The model under review builds one solid part; all positions refer to its coordinate system, in mm. A direction names the side the tool comes from. Coordinates: 2 decimals unless noted, no trailing zeros. Order: outer loops, then holes, each group sorted by start corner. A loop starts at its lowest first (then second) coordinate and runs counter-clockwise, first axis right, second up. Notation, with made-up numbers: M -6.5,58 L 32.5,58 A38 ccw 32.5,97 Z; hole C -12.5,81.25 d7. An arc over 180 degrees is marked long. Write each question's results on one line, items separated by ' | '.
Autodesk Inventor part; units mm, degrees
ref_plane "YZ Plane" through (0, 0, 0) normal (1, 0, 0) x (0, 1, 0)
ref_plane "XZ Plane" through (0, 0, 0) normal (0, 1, 0) x (-1, 0, 0)
ref_plane "XY Plane" through (0, 0, 0) normal (0, 0, 1) x (1, 0, 0)
sketch "Skizze1" plane through (0, 0, 0) normal (0, 0, 1) x (1, 0, 0)
  circle A0 centre (-5, 0) radius 2.15
  circle A1 centre (-5, 0) radius 3.5
  line L0 (-15.4774, 0) -> (15.4774, 0) construction
  line L1 (0, 6.6843) -> (0, -6.6843) construction
  circle A2 centre (5, 0) radius 2.15
  circle A3 centre (5, 0) radius 3.5
  line L2 (-8.5, 3.5) -> (8.5, 3.5)
  line L3 (8.5, 3.5) -> (8.5, -3.5)
  line L4 (8.5, -3.5) -> (-8.5, -3.5)
  line L5 (-8.5, -3.5) -> (-8.5, 3.5)
  line L6 (26, -3.5) -> (-26, -3.5)
  line L7 (-26, -3.5) -> (-26, 3.5)
  line L8 (-26, 3.5) -> (26, 3.5)
  line L9 (26, 3.5) -> (26, -3.5)
  line L10 (26, -3.5) -> (-26, 3.5) construction
  line L11 (-26, -3.5) -> (26, 3.5) construction
  point P0 (0, 0)
  point P1 (0, 0)
  dimension "d0" = 4.3
  dimension "d1" = 7
  dimension "d2" = 10
  dimension "d7" = 52
extrude "Extrusion1" add sketch "Skizze1" along normal blind 12.5 contours A1 | A3
extrude "Extrusion2" add sketch "Skizze1" along normal blind 4
chamfer "Fase1" [suppressed]
fillet "Rundung1" radius 1.5 2 edges at (-26, 0, 4) (26, 0, 4)
properties part number "6_3D-Druck"
1) For pin 1 (3.5 mm diameter, centred on x = -16.5, y = -0.5, fed in from +Z); pin 2 (3.5 mm diameter, centred on x = 5, y = 0, fed in from +Z) (3 decimals); pin 3 (1 mm diameter, centred on y = 2.5, z = 10.5, fed in from -X), all flat-tipped, find the tip position at first contact; note any pin that passes through.
Solutions:
pin 1: z = 4 | pin 2: through | pin 3: x = -7.87
2) To check wall thickness, follow line 1 along Y through (x, z) = (5, 7.25); line 2 along X through (y, z) = (-1.5, 10.25); line 3 along Z through (x, y) = (-16, 3). State the ranges of each line that lie inside material, in increasing order.
Solutions:
line 1: -3.5 to -2.15, 2.15 to 3.5 | line 2: -8.16 to -6.54, -3.46 to -1.84, 1.84 to 3.46, 6.54 to 8.16 | line 3: 0 to 4
3) Take a section at C-C on z = 8. State the section outline as (x, y) points.
Solutions:
outline: C -5,0 d7; C 5,0 d7; hole C -5,0 d4.3; hole C 5,0 d4.3
4) The part is to be moulded in two halves that separate along X. For faces 1 (the cylindrical face through (8.34, -1.05, 8.19)), 2 (the flat face through (0, 0, 4)), 3 (the flat face through (26, 0, 1)), 4 (the cylindrical face through (-25.57, 0.05, 3.55)), say which applies: pulls with the +X half, pulls with the -X half, needs draft (parallel to the pull), parting line crosses it, or undercut.
Solutions:
face 1: undercut | face 2: undercut | face 3: pulls with the +X half | face 4: pulls with the -X half
5) Take a section at B-B on x = 4. State the section outline as (y, z) points, plus the area to 3 significant figures.
Solutions:
outline: M -3.5,0 L -1.9,0 L -1.9,12.5 L -3.35,12.5 L -3.35,4 L -3.5,4 Z; M 1.9,0 L 3.5,0 L 3.5,4 L 3.35,4 L 3.35,12.5 L 1.9,12.5 Z | area: 37.4 mm2
6) Take a section at A-A on y = 0. State the section outline as (x, z) points, plus the area to 3 significant figures.
Solutions:
outline: M -26,0 L -7.15,0 L -7.15,12.5 L -8.5,12.5 L -8.5,4 L -24.5,4 A1.5 ccw -26,2.5 Z; M -2.85,0 L 2.85,0 L 2.85,12.5 L 1.5,12.5 L 1.5,4 L -1.5,4 L -1.5,12.5 L -2.85,12.5 Z; M 7.15,0 L 26,0 L 26,2.5 A1.5 ccw 24.5,4 L 8.5,4 L 8.5,12.5 L 7.15,12.5 Z | area: 219 mm2
7) For faces 5 (the cylindrical face through (-1.767, 1.341, 8.19)), 6 (the flat face through (-7, -2, 12.5)), list the 3-axis set-ups (+Z, -Z, +X, -X, +Y, -Y) from which the entire face can be reached by the end or side of a thin tool; tool diameter is ignored.
Solutions:
face 5: +Z | face 6: +Z, +X, -X, +Y, -Y
8) Take a section at D-D on y = 2.75. State the section outline as (x, z) points, plus the area to 3 significant figures.
Solutions:
outline: M -26,0 L 26,0 L 26,2.5 A1.5 ccw 24.5,4 L 7.17,4 L 7.17,12.5 L 2.83,12.5 L 2.83,4 L -2.83,4 L -2.83,12.5 L -7.17,12.5 L -7.17,4 L -24.5,4 A1.5 ccw -26,2.5 Z | area: 281 mm2
